from build123d import *

# Parameters (mm, degrees)
SKETCH_1_W          = 93
SKETCH_1_H          = 87
SKETCH_1_R          = 1.6
EXTRUDE_1_DEPTH     = 7
SKETCH_3_W          = 93
SKETCH_3_H          = 16
CUT_EXTRUDE_1_DEPTH = 5.5
SKETCH_4_W          = 78.2
SKETCH_4_H          = 51
EXTRUDE_2_DEPTH     = 9
SKETCH_5_W          = 12
SKETCH_5_H          = 12
EXTRUDE_3_DEPTH     = 7
SKETCH_6_R          = 3.35
EXTRUDE_4_DEPTH     = 7.5
SKETCH1_W           = 5.4
SKETCH1_H           = 43
BOSS_EXTRUDE1_DEPTH = 4
SKETCH2_R           = 6
BOSS_EXTRUDE2_DEPTH = 10
SKETCH3_W           = 50
SKETCH3_H           = 4
BOSS_EXTRUDE3_DEPTH = 4.5
SKETCH4_W           = 7.5
SKETCH4_H           = 7
BOSS_EXTRUDE4_DEPTH = 9
SKETCH5_W           = 6
SKETCH5_H           = 6
BOSS_EXTRUDE5_DEPTH = 7


with BuildPart() as part:
    # Эскиз1 → Бобышка-Вытянуть1 (new body)
    with BuildSketch(Plane(origin=(0, 0, 0), x_dir=(1, 0, 0), z_dir=(0, 1, 0))):
        with Locations((46.5, 43.5)):
            Rectangle(SKETCH_1_W, SKETCH_1_H)
        with Locations((3, 84.4)):
            Circle(SKETCH_1_R, mode=Mode.SUBTRACT)
        with Locations((90, 84.4)):
            Circle(SKETCH_1_R, mode=Mode.SUBTRACT)
        with Locations((90, 18.6)):
            Circle(SKETCH_1_R, mode=Mode.SUBTRACT)
        with Locations((3, 18.6)):
            Circle(SKETCH_1_R, mode=Mode.SUBTRACT)
    extrude(amount=EXTRUDE_1_DEPTH)

    # Эскиз3 → Вырез-Вытянуть1 (cut)
    with BuildSketch(Plane(origin=(0, 7, 0), x_dir=(1, 0, 0), z_dir=(0, 1, 0))):
        with Locations((46.5, 8)):
            Rectangle(SKETCH_3_W, SKETCH_3_H)
    extrude(amount=-CUT_EXTRUDE_1_DEPTH, mode=Mode.SUBTRACT)

    # Эскиз4 → Бобышка-Вытянуть2 (add)
    with BuildSketch(Plane(origin=(0, 7, 0), x_dir=(1, 0, 0), z_dir=(0, 1, 0))):
        with Locations((46.5, 52.1)):
            Rectangle(SKETCH_4_W, SKETCH_4_H)
    extrude(amount=EXTRUDE_2_DEPTH)

    # Эскиз5 → Бобышка-Вытянуть3 (add)
    with BuildSketch(Plane(origin=(0, 1.5, 0), x_dir=(1, 0, 0), z_dir=(0, 1, 0))):
        with Locations((83, 8.5)):
            Rectangle(SKETCH_5_W, SKETCH_5_H)
    extrude(amount=EXTRUDE_3_DEPTH)

    # Эскиз6 → Бобышка-Вытянуть4 (add)
    with BuildSketch(Plane(origin=(0, 8.5, 0), x_dir=(1, 0, 0), z_dir=(0, 1, 0))):
        with Locations((83, 8.5)):
            Circle(SKETCH_6_R)
    extrude(amount=EXTRUDE_4_DEPTH)

    # Sketch1 → Boss-Extrude1 (add)
    with BuildSketch(Plane(origin=(0, 7, 0), x_dir=(1, 0, 0), z_dir=(0, 1, 0))):
        with Locations((4.7, 52.1)):
            Rectangle(SKETCH1_W, SKETCH1_H)
    extrude(amount=BOSS_EXTRUDE1_DEPTH)

    # Эскиз9 → Revolve1 (revolve)
    with BuildSketch(Plane.ZY.offset(-83)):
        Polygon((-8.5, 16), (-16, 16), (-16, 18), (-13.5, 31), (-8.5, 31), align=None)
    revolve(axis=Axis((83, 16, -8.5), (0, 1, 0)))

    # Sketch2 → Boss-Extrude2 (add)
    with BuildSketch(Plane(origin=(0, 1.5, 0), x_dir=(1, 0, 0), z_dir=(0, 1, 0))):
        with Locations((65.3, 8)):
            Circle(SKETCH2_R)
    extrude(amount=BOSS_EXTRUDE2_DEPTH)

    # Sketch3 → Boss-Extrude3 (add)
    with BuildSketch(Plane(origin=(0, 7, 0), x_dir=(1, 0, 0), z_dir=(0, 1, 0))):
        with Locations((37, 18)):
            Rectangle(SKETCH3_W, SKETCH3_H)
    extrude(amount=BOSS_EXTRUDE3_DEPTH)

    # Sketch4 → Boss-Extrude4 (add)
    with BuildSketch(Plane(origin=(0, 1.5, 0), x_dir=(1, 0, 0), z_dir=(0, 1, 0))):
        with Locations((9.25, 11.5)):
            Rectangle(SKETCH4_W, SKETCH4_H)
    extrude(amount=BOSS_EXTRUDE4_DEPTH)

    # Sketch5 → Boss-Extrude5 (add)
    with BuildSketch(Plane(origin=(0, 1.5, 0), x_dir=(1, 0, 0), z_dir=(0, 1, 0))):
        with Locations((50, 8.5)):
            Rectangle(SKETCH5_W, SKETCH5_H)
    extrude(amount=BOSS_EXTRUDE5_DEPTH)


solid = part.part
Geometry check sheet. Reference: the model listing, model coordinates, mm. A direction names the side the tool comes from. Round coordinates to 2 decimals unless told otherwise and drop trailing zeros. Order: outer loops, then holes, each group sorted by start corner. A loop starts at its lowest first (then second) coordinate and runs counter-clockwise, first axis right, second up. Notation, with made-up numbers: M 80.25,58 L 85.25,58 A7 ccw 85.25,68 Z; hole C 65,67 d6. An arc over 180 degrees is marked long. Write each question's results on one line, items separated by ' | '. Start each with the question number.
1. Go/stop test with flat-tipped pins: P1, Ø1.5, axis at x = 73.5, y = 13.5, coming from the +Z side; P2, Ø2, axis at y = 9, z = -18.5, coming from the -X side; P3, Ø2, axis at x = 47.5, y = 9.5, coming from the -Z side. Record where each tip stops, or that it passes through.
2. Cross-section at A-A on z = -84.4. Record the boundary of the cut face in (x, y).
3. Material ranges on L1, parallel to Z at x = 3, y = 5; L2, parallel to X at y = 2.25, z = -18.6; L3, parallel to X at y = 2, z = -18, recorded low to high. Write a range as from..to.
4. Set-up check for faces 5 (the face through (37, 11.5, -18)), 6 (the face through (53, 5, -8)), 7 (the face through (5, 11, -52)): record each of +Z, -Z, +X, -X, +Y, -Y from which the full face is reachable in a straight line by a thin tool's end or side.
5. Cross-section at B-B on x = 83. Record the boundary of the cut face in (y, z), plus the area to 3 significant figures.
6. Cross-section at C-C on z = -75. Record the boundary of the cut face in (x, y), plus the area to 3 significant figures.
7. Draft check along Z on faces 1 (the face through (46, 11, -77.6)), 2 (the face through (2, 9, -52)), 3 (the face through (85, 16, -5)), 4 (the face through (53, 7, -78)). Enter one of: pulls with the +Z half, pulls with the -Z half, needs draft (parallel to the pull), parting line crosses it, or undercut.
8. Cross-section at D-D on x = 65.3. Record the boundary of the cut face in (y, z), plus the area to 3 significant figures.
Resolved:
1) P1: z = -26.6 | P2: x = 12 | P3: z = -77.6
2) outline: M 0,0 L 1.4,0 L 1.4,7 L 0,7 Z; M 4.6,0 L 88.4,0 L 88.4,7 L 4.6,7 Z; M 91.6,0 L 93,0 L 93,7 L 91.6,7 Z
3) L1: -87..-86, -82.8..-20.2, -17..-16 | L2: 0..1.4, 4.6..88.4, 91.6..93 | L3: 0..1.52, 4.48..88.52, 91.48..93
4) face 5: +Z, +X, -X, +Y | face 6: +Z, +Y | face 7: +Z, -Z, -X, +Y
5) outline: M 0,-87 L 7,-87 L 7,-77.6 L 16,-77.6 L 16,-26.6 L 7,-26.6 L 7,-16 L 1.5,-16 L 1.5,-14.5 L 8.5,-14.5 L 8.5,-11.85 L 16,-11.85 L 16,-16 L 18,-16 L 31,-13.5 L 31,-3.5 L 18,-1 L 16,-1 L 16,-5.15 L 8.5,-5.15 L 8.5,-2.5 L 1.5,-2.5 L 1.5,0 L 0,0 Z | area: 1,310 mm2
6) outline: M 0,0 L 93,0 L 93,7 L 85.6,7 L 85.6,16 L 7.4,16 L 7.4,7 L 0,7 Z | area: 1,350 mm2
7) face 1: pulls with the -Z half | face 2: needs draft | face 3: undercut | face 4: undercut
8) outline: M 0,-87 L 7,-87 L 7,-77.6 L 16,-77.6 L 16,-26.6 L 7,-26.6 L 7,-16 L 1.5,-16 L 1.5,-14 L 11.5,-14 L 11.5,-2 L 1.5,-2 L 1.5,0 L 0,0 Z | area: 1,100 mm2
